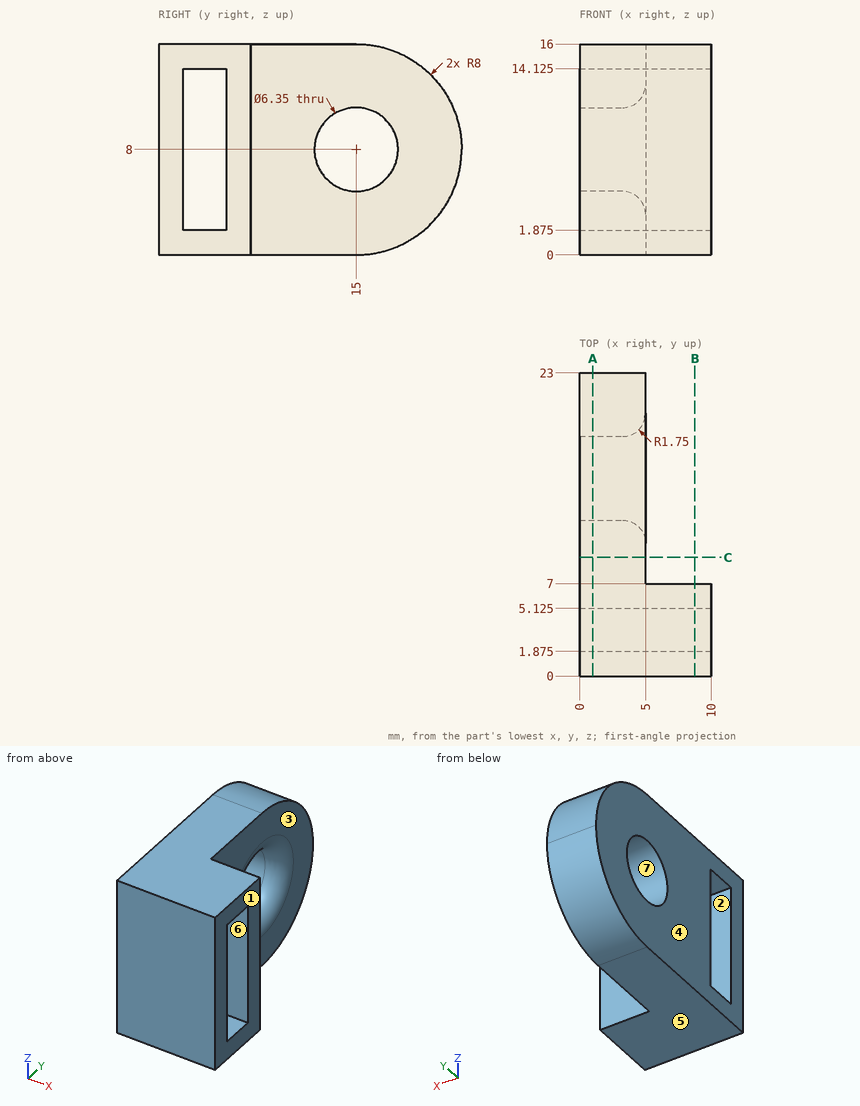
Drawing for the job (mm, zero at the part's lowest x, y, z). A direction names the side the tool comes from. Round coordinates to 2 decimals unless told otherwise and drop trailing zeros. Write each loop counter-clockwise with the first axis right and the second up, starting at its lowest first coordinate (ties: lowest second). Pieces come first, ordered by that corner, then holes. Notation, with made-up numbers: M 5.5,58 L 22.5,58 A19 cw 22.5,75 Z; hole C 79.5,72.25 d5. An arc over 180 degrees is marked long. Answer in a Markdown table with one row per item.
1. Which spindle directions (+Z, -Z, +X, -X, +Y, -Y) get a long thin tool onto all of the face, cutting with end or side? Do the marked faces 1, 2 and 3. Say none if no direction does.
Geometry check:
| item | result |
|---|---|
| face 1 | +Z, -Z, +X, +Y, -Y |
| face 2 | +X, -X |
| face 3 | +Z, -Z, +X, +Y |
2. Saw through at B-B (x = 8.75). List the corners of the cut face in (y, z) (1 decimal).
Geometry check:
| item | result |
|---|---|
| outline | M 0,0 L 7,0 L 7,16 L 0,16 Z; hole M 1.9,1.9 L 5.1,1.9 L 5.1,14.1 L 1.9,14.1 Z |
3. Saw through at C-C (y = 9). List the corners of the cut face in (x, z).
Geometry check:
| item | result |
|---|---|
| outline | M 0,0 L 5,0 L 5,16 L 0,16 Z |
4. Probe L1, parallel to Y at x = 1.75, z = 8 (1 decimal); L2, parallel to Y at x = 7.5, z = 12.5 (1 decimal); L3, parallel to Z at x = 8, y = 3.25 (1 decimal). List the from-to ranges inside material, lowest first. Write a range as [from, to].
Geometry check:
| item | result |
|---|---|
| L1 | [0, 1.9], [5.1, 11.8], [18.2, 23] |
| L2 | [0, 1.9], [5.1, 7] |
| L3 | [0, 1.9], [14.1, 16] |
5. Mould opens along Z. For the marked faces 4, 5, 6 and 7 say: +Z half, -Z half, draft (parallel to the pull), parting line (faces both ways), or undercut.
Geometry check:
| item | result |
|---|---|
| face 4 | draft |
| face 5 | -Z half |
| face 6 | undercut |
| face 7 | undercut |
6. Saw through at A-A (x = 1). State how many separate pieces and enclosed holes the cut face has, and give its area (3 significant figures).
Geometry check:
| item | result |
|---|---|
| separate pieces | 1 |
| enclosed holes | 2 |
| area | 269 mm2 |
7. Flat gauge pins, fed straight in: P1, Ø5.5, axis at x = 8, z = 11.5, coming from the +Y side; P2, Ø2, axis at x = 2, z = 9, coming from the -Y side. Where does each tip first touch, or does it go through?
Geometry check:
| item | result |
|---|---|
| P1 | y = 7 |
| P2 | y = 0 |
